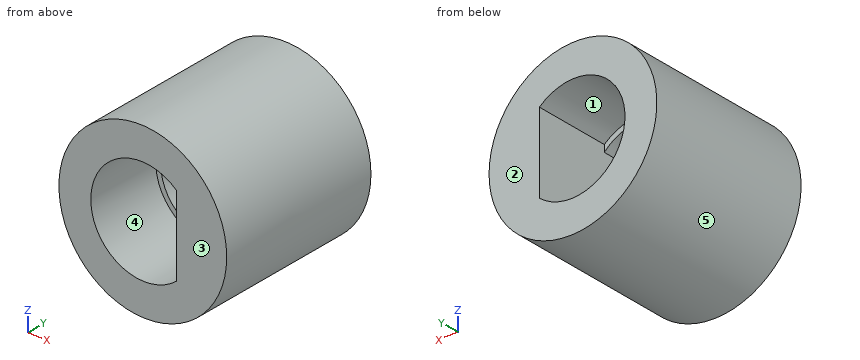
```python
from build123d import *
from build123d.topology import SkipClean

# Parameters (mm, degrees)
EXTRUDE_1_DEPTH      = 0.25
EXTRUDE_1_DEPTH_BACK = 0.25
SKETCH_1_R           = 2.5
SKETCH_1_R_2         = 1.4
EXTRUDE_START        = -2.5
EXTRUDE_2_OUTLINE_R  = 2.5
EXTRUDE_2_DEPTH      = 5


# Read off the part's stored shape, not the designer's step: the extrude step
with BuildPart() as part:
    # Sketch 1 → Extrude 1 (new, two sides: drawn at the far end of the back side and taken through both)
    with BuildSketch(Plane(origin=(0, 0, 0), x_dir=(1, 0, 0), z_dir=(0, 1, 0)).offset(-EXTRUDE_1_DEPTH_BACK)):
        with Locations(Location((0, 0, 0), (0, 0, 270))):
            Circle(SKETCH_1_R)
        with Locations(Location((0, 0, 0), (0, 0, 270))):
            Circle(SKETCH_1_R_2, mode=Mode.SUBTRACT)
    extrude(amount=EXTRUDE_1_DEPTH + EXTRUDE_1_DEPTH_BACK)

    # Extrude 2 outline → Extrude 2 (add)
    with SkipClean():  # the faces are left unmerged after this step: merging them gives an invalid solid
        with BuildSketch(Plane(origin=(0, 0, 0), x_dir=(1, 0, 0), z_dir=(0, 1, 0)).offset(EXTRUDE_START)):
            Circle(EXTRUDE_2_OUTLINE_R)
            with BuildLine():
                ThreePointArc((1, -1.184271928), (-1.55, 0), (1, 1.184271928))
                Line((1, 1.184271928), (1, -1.184271928))
            make_face(mode=Mode.SUBTRACT)
        extrude(amount=EXTRUDE_2_DEPTH)
    add(part.part.scale(1), mode=Mode.REPLACE)  # the faces are merged on a copy


solid = part.part
```
Geometry check sheet. Reference: the model listing, model coordinates, mm. Face numbers are marked on the shaded views. A direction names the side the tool comes from. Round coordinates to 2 decimals unless told otherwise and drop trailing zeros. Loops run counter-clockwise (first coordinate to the right, second up) from the corner with the lowest first, then second, coordinate; pieces in that order, holes last. Notation, with made-up numbers: (-20.75, 80.25) - (-4.75, 80.25) arc R17 ccw to (-4.75, 113.25) - close; hole circle Ø2 at (33.25, 82.25). An arc over 180 degrees is marked (long way). Use a Markdown table: item, result.
Q1. Access from +Z, -Z, +X, -X, +Y, -Y to the whole of each face (thin tool, end or side, straight path). Record for the marked faces 1 and 2.
Solutions:
| item | result |
|---|---|
| face 1 | +Y |
| face 2 | +Z, -Z, +X, -X, +Y |
Q2. Go/stop test with flat-tipped pins: P1, Ø2, axis at x = -2, y = 1.5, coming from the +Z side; P2, Ø1.9, axis at x = 0, z = 0, coming from the +Y side; P3, Ø0.7, axis at y = -0.5, z = -0.5, coming from the -X side. Record where each tip stops, or that it passes through.
Solutions:
| item | result |
|---|---|
| P1 | stops at z = 2.29 |
| P2 | passes through |
| P3 | stops at x = -2.5 |
Q3. Cross-section at A-A on x = -0.15. Record the cut outline in (y, z), plus the area to 3 significant figures.
Solutions:
| item | result |
|---|---|
| outline | (-2.5, -2.5) - (2.5, -2.5) - (2.5, -1.54) - (0.25, -1.54) - (0.25, -1.39) - (-0.25, -1.39) - (-0.25, -1.54) - (-2.5, -1.54) - close; (-2.5, 1.54) - (-0.25, 1.54) - (-0.25, 1.39) - (0.25, 1.39) - (0.25, 1.54) - (2.5, 1.54) - (2.5, 2.5) - (-2.5, 2.5) - close |
| area | 9.68 mm2 |
Q4. Material ranges on line 1 (Z direction, x = 0, y = -1.3); line 2 (Z direction, x = 0, y = 0.1); line 3 (X direction, y = 0.3, z = -1.35), recorded low to high.
Solutions:
| item | result |
|---|---|
| line 1 | z = -2.5 to -1.55, 1.55 to 2.5 |
| line 2 | z = -2.5 to -1.4, 1.4 to 2.5 |
| line 3 | x = -2.1 to -0.76, 0.76 to 2.1 |
Q5. Draft check along X on the marked faces 3, 4 and 5. Enter one of: released by +X, released by -X, zero draft, split by the parting line, or undercut.
Solutions:
| item | result |
|---|---|
| face 3 | zero draft |
| face 4 | undercut |
| face 5 | split by the parting line |
Q6. Cross-section at B-B on y = 1.25. Record the cut outline in (x, z).
Solutions:
| item | result |
|---|---|
| outline | circle Ø5 at (0, 0); hole (1, -1.18) - (1, 1.18) arc R1.55 ccw (long way) to start |
